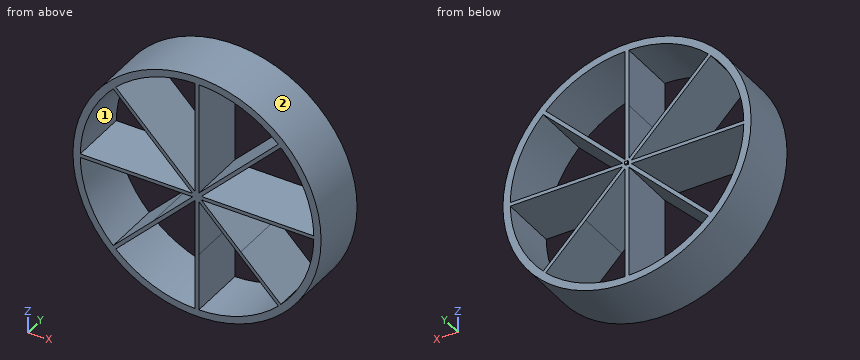
Autodesk Inventor part; units mm, degrees
ref_plane "YZ Plane" through (0, 0, 0) normal (1, 0, 0) x (0, 1, 0)
ref_plane "XZ Plane" through (0, 0, 0) normal (0, 1, 0) x (-1, 0, 0)
ref_plane "XY Plane" through (0, 0, 0) normal (0, 0, 1) x (1, 0, 0)
sketch "Sketch1" plane through (0, 0, 0) normal (0, 1, 0) x (-1, 0, 0)
  circle A0 centre (0, 0) radius 50.8
  circle A1 centre (0, 0) radius 53.975
  dimension "d0" = 101.6
  dimension "d1" = 107.95
extrude "Extrusion1" add sketch "Sketch1" along normal blind 25.4 contours A0 | A1
sketch "Sketch2" plane through (0, 25.4, 0) normal (0, 1, 0) x (1, 0, 0)
  circle A0 centre (0, 0) radius 50.8
  dimension "d4" = 101.6
extrude "Extrusion2" cut sketch "Sketch2" against normal blind 22.225
sketch "Sketch3" plane through (0, 3.175, 0) normal (0, 1, 0) x (1, 0, 0)
  line L0 (-0.7937, 25.8929) -> (0.7937, -25.8929) construction
  line L1 (0.7937, 25.8929) -> (-0.7937, -25.8929) construction
  circle A0 centre (0, 0) radius 53.975
  line L2 (-0.7937, 1.9214) -> (-17.916, 19.0437)
  line L3 (0.7938, 1.9213) -> (17.9468, 19.0743)
  line L4 (0.0335, 1.0941) -> (-0.0357, 1.1633)
  line L5 (0.7937, -1.9112) -> (17.9683, -19.0858)
  line L6 (0.0332, -1.0843) -> (-0.0353, -1.1529)
  line L7 (-0.7938, -1.9113) -> (-17.8495, -18.967)
  line L8 (-0.0332, -1.0842) -> (0.0353, -1.1528)
  line L9 (-0.0335, 1.094) -> (0.0357, 1.1632)
  line L10 (-25.8929, 0.7937) -> (-0.7937, 0.0243) construction
  line L11 (0, 0) -> (25.8929, -0.7937) construction
  line L12 (-25.8929, 0.7937) -> (-1.9112, 0.7937)
  line L13 (-0.0243, 0.7937) -> (0.0243, 0.7937)
  line L14 (1.9113, 0.7937) -> (25.8929, 0.7937)
  line L15 (-0.7937, 1.9214) -> (-0.7937, 25.8929)
  line L16 (-0.7937, -25.8929) -> (-0.7938, -1.9113)
  line L17 (-0.7937, -0.0243) -> (-0.7937, 0.0243)
  line L18 (-1.9213, -0.7937) -> (-25.8929, -0.7937)
  line L19 (25.8929, -0.7937) -> (1.9214, -0.7937)
  line L20 (0.0243, -0.7937) -> (-0.0243, -0.7937)
  line L21 (0.7937, -1.9112) -> (0.7937, -25.8929)
  line L22 (0.7937, 25.8929) -> (0.7938, 1.9213)
  line L23 (0.7937, 0.0243) -> (0.7937, -0.0243)
  line L24 (25.8929, 0.7937) -> (0, 0) construction
  line L25 (-0.7937, -0.0243) -> (-25.8929, -0.7937) construction
  line L26 (19.0693, 17.9518) -> (1.9113, 0.7937)
  line L27 (1.1529, 0.0353) -> (1.0843, -0.0332)
  line L28 (19.0909, -17.9632) -> (1.9214, -0.7937)
  line L29 (1.1633, -0.0357) -> (1.0941, 0.0335)
  line L30 (-18.9721, -17.8445) -> (-1.9213, -0.7937)
  line L31 (-1.1632, -0.0357) -> (-1.094, 0.0335)
  line L32 (-19.0386, 17.9211) -> (-1.9112, 0.7937)
  line L33 (-1.1528, 0.0353) -> (-1.0842, -0.0332)
  line L34 (0.7937, 25.8929) -> (0.7937, 52.3915)
  line L35 (0.7937, 52.3915) -> (-0.7937, 52.3915)
  line L36 (-0.7937, 52.3915) -> (-0.7937, 25.8929)
  line L37 (-19.0386, 17.9211) -> (-38.1124, 36.995)
  line L38 (-38.1124, 36.995) -> (-36.9899, 38.1176)
  line L39 (-36.9899, 38.1176) -> (-17.916, 19.0437)
  line L40 (-25.8929, -0.7937) -> (-52.6358, -0.7937)
  line L41 (-52.6358, -0.7937) -> (-52.6358, 0.7937)
  line L42 (-52.6358, 0.7937) -> (-25.8929, 0.7937)
  line L43 (-17.8495, -18.967) -> (-36.1442, -37.2617)
  line L44 (-36.1442, -37.2617) -> (-37.2668, -36.1392)
  line L45 (-37.2668, -36.1392) -> (-18.9721, -17.8445)
  line L46 (0.7937, -25.8929) -> (0.7937, -52.94)
  line L47 (0.7937, -52.94) -> (-0.7937, -52.94)
  line L48 (-0.7937, -52.94) -> (-0.7937, -25.8929)
  line L49 (17.9683, -19.0858) -> (36.3915, -37.509)
  line L50 (36.3915, -37.509) -> (37.5141, -36.3864)
  line L51 (37.5141, -36.3864) -> (19.0909, -17.9632)
  line L52 (25.8929, -0.7937) -> (52.8491, -0.7937)
  line L53 (52.8491, -0.7937) -> (52.8491, 0.7937)
  line L54 (52.8491, 0.7937) -> (25.8929, 0.7937)
  line L55 (19.0693, 17.9518) -> (38.1125, 36.995)
  line L56 (38.1125, 36.995) -> (36.99, 38.1176)
  line L57 (36.99, 38.1176) -> (17.9468, 19.0743)
  point P0 (0.7938, -0.7937)
  point P1 (-0.7938, 0.7937)
  point P2 (-0.7938, -0.7937)
  point P3 (0.7938, 0.7937)
  dimension "d7" = 1.5875
  dimension "d8" = 1.5875
  dimension "d9" = 1.5875
  dimension "d13" = 1.5875
sketch "Sketch5" plane through (0, 3.175, 0) normal (0, 1, 0) x (1, 0, 0)
  circle A0 centre (0, 0) radius 50.8
  circle A1 centre (0, 0) radius 50.8
  circle A2 centre (0, 0) radius 50.8
  circle A3 centre (0, 0) radius 50.8
  circle A4 centre (0, 0) radius 50.8
  circle A5 centre (0, 0) radius 50.8
  circle A6 centre (0, 0) radius 50.8
  circle A7 centre (0, 0) radius 50.8
extrude "Extrusion5" cut sketch "Sketch5" against normal blind 22.225
sketch "Sketch6" plane through (0, 25.4, 0) normal (0, 1, 0) x (1, 0, 0)
  line L0 (0.635, 0.635) -> (-0.635, 0.635)
  line L1 (-0.635, 0.635) -> (-0.635, -0.635)
  line L2 (-0.635, -0.635) -> (0.635, -0.635)
  line L3 (0.635, -0.635) -> (0.635, 0.635)
  line L4 (0.635, 0.635) -> (-0.635, -0.635) construction
  line L5 (-0.635, 0.635) -> (0.635, -0.635) construction
  point P0 (0, 0)
  dimension "d21" = 1.27
  dimension "d22" = 1.27
extrude "Extrusion6" add sketch "Sketch6" along normal blind 0.635
extrude "Extrusion7" add sketch "Sketch3" along normal blind 22.225 and the other way blind 3.175 contours L15 L36 L35 L34 L22 L3 L57 L56 L55 L26 L14 L54 L53 L52 L19 L28 L51 L50 L49 L5 L21 L46 L47 L48 L16 L7 L43 L44 L45 L30 L18 L40 L41 L42 L12 L32 L37 L38 L39 L2
properties part number "FeedWheel"
For this review, take the finished solid that the model builds, in its own axes (mm). Face numbers are marked on the shaded views. Coordinates: 2 decimals unless noted, no trailing zeros. Write each loop counter-clockwise with the first axis right and the second up, starting at its lowest first coordinate (ties: lowest second). Pieces come first, ordered by that corner, then holes.
(1) Add section D-D on z = -42. Give the boundary of the cut face in (x, y).
(2) Add section A-A on y = 2.75. Count the separate pieces of the cut face and the enclosed holes in it, then the cut area to 3 significant figures.
(3) Wall thickness on probe 1 along X at (y, z) = (6.25, -39.5); probe 2 along Z at (x, y) = (18.5, 23); probe 3 along X at (y, z) = (18.5, 8): over which ranges is each line inside the solid? List them lowest first.
(4) For pin 1 Ø1.5 at (x, y) = (37.5, 23.5) entering from +Z; pin 2 Ø0.7 at (y, z) = (26, 0) entering from -X (3 decimals); pin 3 Ø7.5 at (x, y) = (-27, 8) entering from +Z, all flat-tipped, find the tip position at first contact; note any pin that passes through.
(5) Add section B-B on x = 46. Give the boundary of the cut face in (y, z), then the cut area to 3 significant figures.
(6) The part is to be moulded in two halves that separate along Z. For the marked faces 1 and 2, say which applies: +Z half, -Z half, draft (parallel to the pull), parting line (faces both ways), or undercut.
(7) Add section C-C on x = 8. Give the boundary of the cut face in (y, z), then the cut area to 3 significant figures.
Answer sheet:
1. outline: (-33.9, 0) - (-28.58, 0) - (-28.58, 25.4) - (-33.9, 25.4) - close; (-0.79, 0) - (0.79, 0) - (0.79, 25.4) - (-0.79, 25.4) - close; (28.58, 0) - (33.9, 0) - (33.9, 25.4) - (28.58, 25.4) - close
2. separate pieces: 1
2. enclosed holes: 8
2. area: 1,680 mm2
3. probe 1: x = -36.78 to -31.94, -0.79 to 0.79, 31.94 to 36.78
3. probe 2: z = -50.71 to -47.31, -19.63 to -17.38, -0.79 to 0.79, 17.37 to 19.62, 47.31 to 50.71
3. probe 3: x = -53.38 to -50.17, -9.13 to -6.88, -0.79 to 0.79, 6.88 to 9.13, 50.17 to 53.38
4. pin 1: stops at z = 39.53
4. pin 2: stops at x = -0.635
4. pin 3: stops at z = 48.71
5. outline: (0, -28.24) - (25.4, -28.24) - (25.4, -21.56) - (0, -21.56) - close; (0, -0.79) - (25.4, -0.79) - (25.4, 0.79) - (0, 0.79) - close; (0, 21.56) - (25.4, 21.56) - (25.4, 28.24) - (0, 28.24) - close
5. area: 380 mm2
6. face 1: undercut
6. face 2: parting line
7. outline: (0, -53.38) - (25.4, -53.38) - (25.4, -50.17) - (0, -50.17) - close; (0, -9.13) - (25.4, -9.13) - (25.4, -6.88) - (0, -6.88) - close; (0, -0.79) - (25.4, -0.79) - (25.4, 0.79) - (0, 0.79) - close; (0, 6.87) - (25.4, 6.87) - (25.4, 9.12) - (0, 9.12) - close; (0, 50.17) - (25.4, 50.17) - (25.4, 53.38) - (0, 53.38) - close
7. area: 318 mm2
